Geometry check sheet. Reference: the model listing, model coordinates, mm. A direction names the side the tool comes from. Coordinates: 2 decimals unless noted, no trailing zeros. Write each loop counter-clockwise with the first axis right and the second up, starting at its lowest first coordinate (ties: lowest second). Pieces come first, ordered by that corner, then holes. Notation, with made-up numbers: (-17, 59.25) -> (-3, 59.25) arc R30 ccw to (-3, 93.25) -> close; hole circle Ø9 at (26, -26). An arc over 180 degrees is marked (long way). Answer in a Markdown table with one row per item. Add a question column.
Q1. Thickness scan on line 1 (Z direction, x = 8, y = 16); line 2 (X direction, y = 11.5, z = -31); line 3 (Y direction, x = 19, z = -17). Record the ranges inside material, lowest first.
Q2. Section check D-D, the plane z = -36. Record the boundary of the cut face in (x, y), and give its area (3 significant figures).
Q3. Section check C-C, the plane y = 12. Record the boundary of the cut face in (x, z), and give its area (3 significant figures).
Q4. Release check for a two-part mould opening along X. For faces 1 (the face through (3.077, 15, -32)), 2 (the face through (28, 10, -27)), 3 (the face through (2.577, 15, -32)) record: pulls with the +X half, pulls with the -X half, needs draft (parallel to the pull), parting line crosses it, or undercut.
Q5. Section check B-B, the plane x = 12. Record the boundary of the cut face in (y, z).
Q6. Gauge pin test, flat end, axial feed: P1, Ø15, axis at x = 24.5, z = -26, coming from the +Y side. Record the tip position at first contact, or that the pin passes through.
Q7. Tool access check on faces 4 (the face through (53.877, 15, -32)), 5 (the face through (54.377, 15, -32)). Record the directions out of +Z, -Z, +X, -X, +Y, -Y that give a thin tool (end or side, any length) a straight path to the whole face; none if there is none.
Q8. Section check A-A, the plane z = -55. Record the boundary of the cut face in (x, y), and give its area (3 significant figures).
```python
from build123d import *

# Parameters (mm, degrees)
SKETCH2_W           = 51.8
SKETCH2_H           = 51.8
BOSS_EXTRUDE1_DEPTH = 20
SKETCH3_W           = 50.8
SKETCH3_H           = 50.8
CUT_EXTRUDE1_DEPTH  = 19.5
SKETCH4_W           = 8.13
SKETCH4_H           = 8.13
SKETCH4_W_2         = 8.128
SKETCH4_H_2         = 8.128
SKETCH4_W_3         = 10.368
SKETCH4_H_3         = 3.05
SKETCH4_R           = 0.25
CUT_EXTRUDE2_DEPTH  = 21
SKETCH4_3_R         = 0.25
CUT_EXTRUDE3_DEPTH  = 19.5
SKETCH5_W           = 51.8
SKETCH5_H           = 10
CUT_EXTRUDE4_DEPTH  = 52.8
SKETCH6_R           = 0.25
CUT_EXTRUDE8_DEPTH  = 2


with BuildPart() as part:
    # Sketch2 → Boss-Extrude1 (new body)
    with BuildSketch(Plane(origin=(0, 10, 0), x_dir=(1, 0, 0), z_dir=(0, 1, 0))):
        with Locations((28.476627116, 32.676299595)):
            Rectangle(SKETCH2_W, SKETCH2_H)
    extrude(amount=BOSS_EXTRUDE1_DEPTH)

    # Sketch3 → Cut-Extrude1 (cut)
    with BuildSketch(Plane(origin=(0, 30, 0), x_dir=(1, 0, 0), z_dir=(0, 1, 0))):
        with Locations((28.476627116, 32.676299595)):
            Rectangle(SKETCH3_W, SKETCH3_H)
    extrude(amount=-CUT_EXTRUDE1_DEPTH, mode=Mode.SUBTRACT)

    # Sketch4 → Cut-Extrude2 (cut, through all)
    with BuildSketch(Plane.XZ.offset(-10)):
        with Locations((42.061627116, -53.511299595)):
            Rectangle(SKETCH4_W, SKETCH4_H)
        with Locations((28.475627116, -53.511299595)):
            Rectangle(SKETCH4_W, SKETCH4_H)
        with Locations((14.890627116, -53.512299595)):
            Rectangle(SKETCH4_W_2, SKETCH4_H_2)
        with Locations((28.492627116, -32.551299595)):
            Rectangle(SKETCH4_W_3, SKETCH4_H_3)
        with Locations((32.768731714, -23.235629349)):
            Circle(SKETCH4_R)
        with Locations((32.111104012, -24.757567746)):
            Circle(SKETCH4_R)
        with Locations((30.175799631, -25.584299714)):
            Circle(SKETCH4_R)
        with Locations((30.68311243, -23.742942148)):
            Circle(SKETCH4_R)
        with Locations((29.340042817, -24.53053501)):
            Circle(SKETCH4_R)
        with Locations((27.613211416, -24.53053501)):
            Circle(SKETCH4_R)
        with Locations((26.777454602, -25.584299714)):
            Circle(SKETCH4_R)
        with Locations((29.340042817, -20.377813869)):
            Circle(SKETCH4_R)
        with Locations((31.547423124, -20.377813869)):
            Circle(SKETCH4_R)
        with Locations((31.547423124, -22.183425025)):
            Circle(SKETCH4_R)
        with Locations((26.270141803, -23.742942148)):
            Circle(SKETCH4_R)
        with Locations((24.842150221, -24.757567746)):
            Circle(SKETCH4_R)
        with Locations((24.184522519, -23.235629349)):
            Circle(SKETCH4_R)
        with Locations((25.405831109, -22.183425025)):
            Circle(SKETCH4_R)
        with Locations((25.405831109, -20.377813869)):
            Circle(SKETCH4_R)
        with Locations((27.613211416, -22.183425025)):
            Circle(SKETCH4_R)
        with Locations((29.340042817, -22.183425025)):
            Circle(SKETCH4_R)
        with Locations((30.68311243, -18.818296747)):
            Circle(SKETCH4_R)
        with Locations((32.111104012, -17.803671149)):
            Circle(SKETCH4_R)
        with Locations((29.340042817, -18.030703885)):
            Circle(SKETCH4_R)
        with Locations((30.175799631, -16.97693918)):
            Circle(SKETCH4_R)
        with Locations((26.777454602, -16.97693918)):
            Circle(SKETCH4_R)
        with Locations((27.613211416, -18.030703885)):
            Circle(SKETCH4_R)
        with Locations((26.270141803, -18.818296747)):
            Circle(SKETCH4_R)
        with Locations((24.842150221, -17.803671149)):
            Circle(SKETCH4_R)
        with Locations((24.184522519, -19.325609546)):
            Circle(SKETCH4_R)
    extrude(amount=-CUT_EXTRUDE2_DEPTH, mode=Mode.SUBTRACT)

    # Sketch4<3> → Cut-Extrude3 (cut)
    with BuildSketch(Plane.XZ.offset(-10)):
        with Locations((32.768731714, -19.325609546)):
            Circle(SKETCH4_3_R)
        with Locations((27.613211416, -20.377813869)):
            Circle(SKETCH4_3_R)
    extrude(amount=-CUT_EXTRUDE3_DEPTH, mode=Mode.SUBTRACT)

    # Sketch5 → Cut-Extrude4 (cut, through all)
    with BuildSketch(Plane(origin=(0, 0, -58.576299595), x_dir=(-1, 0, 0), z_dir=(0, 0, -1))):
        with Locations((-28.476627116, 25)):
            Rectangle(SKETCH5_W, SKETCH5_H)
    extrude(amount=-CUT_EXTRUDE4_DEPTH, mode=Mode.SUBTRACT)

    # Sketch6 → Cut-Extrude8 (cut)
    with BuildSketch(Plane(origin=(0, 20, 0), x_dir=(1, 0, 0), z_dir=(0, 1, 0))):
        with Locations((2.852996887, 58.299929824)):
            Circle(SKETCH6_R)
        with Locations((54.100257345, 58.299929824)):
            Circle(SKETCH6_R)
        with Locations((54.100257345, 7.052669366)):
            Circle(SKETCH6_R)
        with Locations((2.852996887, 7.052669366)):
            Circle(SKETCH6_R)
    extrude(amount=-CUT_EXTRUDE8_DEPTH, mode=Mode.SUBTRACT)


solid = part.part
```
Calculated:
| question | item | result |
|---|---|---|
| 1 | line 1 | z = -58.58 to -58.08, -7.28 to -6.78 |
| 1 | line 2 | x = 2.58 to 3.08, 53.88 to 54.38 |
| 1 | line 3 | y = 10 to 10.5 |
| 2 | outline | (2.58, 10) -> (54.38, 10) -> (54.38, 20) -> (53.88, 20) -> (53.88, 10.5) -> (3.08, 10.5) -> (3.08, 20) -> (2.58, 20) -> close |
| 2 | area | 35.4 mm² |
| 3 | outline | (2.58, -58.58) -> (54.38, -58.58) -> (54.38, -6.78) -> (2.58, -6.78) -> close; hole (3.08, -58.08) -> (53.88, -58.08) -> (53.88, -7.28) -> (3.08, -7.28) -> close |
| 3 | area | 103 mm² |
| 4 | face 1 | undercut |
| 4 | face 2 | needs draft |
| 4 | face 3 | pulls with the -X half |
| 5 | outline | (10, -58.58) -> (20, -58.58) -> (20, -58.08) -> (10.5, -58.08) -> (10.5, -57.58) -> (10, -57.58) -> close; (10, -49.45) -> (10.5, -49.45) -> (10.5, -7.28) -> (20, -7.28) -> (20, -6.78) -> (10, -6.78) -> close |
| 6 | P1 | stops at y = 10.5 |
| 7 | face 4 | +Y |
| 7 | face 5 | +Z, -Z, +X, +Y, -Y |
| 8 | outline | (2.58, 10) -> (10.83, 10) -> (10.83, 10.5) -> (3.08, 10.5) -> (3.08, 20) -> (2.58, 20) -> close; (18.95, 10) -> (24.41, 10) -> (24.41, 10.5) -> (18.95, 10.5) -> close; (32.54, 10) -> (38, 10) -> (38, 10.5) -> (32.54, 10.5) -> close; (46.13, 10) -> (54.38, 10) -> (54.38, 20) -> (53.88, 20) -> (53.88, 10.5) -> (46.13, 10.5) -> close |
| 8 | area | 23.2 mm² |
